Read the model definition and answer for the solid it produces. Units are mm, in the model's axes. Face numbers are marked on the shaded views. A direction names the side the tool comes from. Give positions to 0.01 mm unless a question says otherwise; leave off trailing zeros. Order: outer loops, then holes, each group sorted by start corner. A loop starts at its lowest first (then second) coordinate and runs counter-clockwise, first axis right, second up.
Autodesk Inventor part; units mm, degrees
ref_plane "Work Plane1" through (-2.5, 0, 0) normal (1, 0, 0) x (0, 1, 0)
ref_plane "XZ Plane" through (0, 0, 0) normal (0, 1, 0) x (-1, 0, 0)
ref_plane "XY Plane" through (0, 0, 0) normal (0, 0, 1) x (1, 0, 0)
sketch "Sketch1" plane through (0, 0, 0) normal (0, 0, 1) x (1, 0, 0)
  circle A0 centre (0, 0) radius 2
  circle A1 centre (0, 0) radius 6
  dimension "d0" = 4
  dimension "d1" = 12
extrude "Extrusion1" add sketch "Sketch1" along normal blind 5
ref_plane "Work Plane1" through (-2.5, 0, 0) normal (1, 0, 0) x (0, 1, 0)
sketch "Sketch5" plane through (-2.5, 0, 0) normal (1, 0, 0) x (0, 1, 0)
  line L0 (2.5, 0) -> (-2.5, 0)
  line L1 (-2.5, 0) -> (-2.5, 5)
  line L2 (-2.5, 5) -> (2.5, 5)
  line L3 (2.5, 5) -> (2.5, 0)
  point P0 (0, 0)
  point P1 (0, 0)
  dimension "d5" = 5
  dimension "d6" = 5
extrude "Extrusion2" add sketch "Sketch5" against normal blind 6
sketch "Sketch7" plane through (-8.5, 0, 0) normal (-1, 0, 0) x (0, 0, 1)
  line L0 (0, 2.5) -> (0, -2.5)
  line L1 (0, -2.5) -> (5, -2.5)
  line L2 (5, -2.5) -> (5, 2.5)
  line L3 (5, 2.5) -> (0, 2.5)
  point P0 (0, 0)
extrude "Extrusion3" add sketch "Sketch7" along normal blind 17
sketch "Sketch8" plane through (0, 0, 5) normal (0, 0, 1) x (1, 0, 0)
  line L0 (-25.5, 5) -> (-25.5, -5)
  line L1 (-25.5, -2.5) -> (-25.5, 2.5)
  line L2 (-6.5, 3.5) -> (-6.5, -3.5)
  arc A0 (-25.5, 5) -> (-6.5, 3.5) centre (7.5988, 303.1685) ccw
  arc A1 (-6.5, -3.5) -> (-25.5, -5) centre (7.5988, -303.1685) ccw
  point P0 (0, 0)
  point P1 (-25.5, 0)
  point P2 (-25.5, 0)
  point P3 (-6.5, 0)
  dimension "d11" = 10
  dimension "d12" = 7
  dimension "d13" = 6.5
  dimension "d14" = 300
  dimension "d15" = 300
extrude "Extrusion4" add sketch "Sketch8" against normal blind 6 and the other way blind 1
sketch "Sketch9" plane through (-5.4544, 2.5, 5) normal (0, 1, 0) x (1, 0, 0)
  line L0 (-20.0456, 7.5) -> (-20.0456, -2.5) construction
  line L1 (-20.0456, -1) -> (-20.0456, 6)
  line L2 (-1.0456, 6) -> (-1.0456, -1)
  arc A0 (-20.0456, 7.5) -> (-1.0456, 6) centre (13.0532, 305.6685) ccw
  arc A1 (-1.0456, -1) -> (-20.0456, -2.5) centre (13.0532, -300.6685) ccw
  line L3 (-1.0456, 6) -> (-1.0456, -1)
  line L4 (-20.0456, 6) -> (-1.0456, 6)
  line L5 (-20.0456, -1) -> (-1.0456, -1)
  line L6 (-20.0456, 6) -> (-20.0456, 7.5)
  line L7 (-20.0456, -2.5) -> (-20.0456, -1)
  point P0 (5.4544, 5)
  point P1 (-20.0456, 2.5)
  dimension "d20" = 10
  dimension "d21" = 300
  dimension "d22" = 300
extrude "Extrusion5" add sketch "Sketch9" along normal blind 2.5 and the other way blind 7.5 contours L5 A1 L7 | L6 A0 L4
sketch "Sketch10" plane through (-25.5, 5, -1) normal (0, 0, 1) x (1, 0, 0)
  arc A0 (0, 0) -> (19, -1.5) centre (33.0988, 298.1685) ccw
  line L0 (19, -1.5) -> (19, 0)
  line L1 (0, 0) -> (19, 0)
  arc A1 (19, -8.5) -> (0, -10) centre (33.0988, -308.1685) ccw
  line L2 (19, -10) -> (0, -10)
  line L3 (19, -10) -> (19, -8.5)
  point P0 (25.5, -5)
extrude "Extrusion6" cut sketch "Sketch10" along normal through all both and the other way through all
fillet "Fillet1" radius 2 4 edges at (-16.0467, 4.1018, 6.6018) (-16.0467, 4.1018, -1.6018) (-16.0467, -4.1018, 6.6018) (-16.0467, -4.1018, -1.6018)
sketch "Sketch11" plane through (-25.5, 0, 0) normal (-1, 0, 0) x (0, 0, 1)
  circle A0 centre (2.5, 0) radius 1.5
  line L0 (5.5122, 5) -> (-0.5122, 5)
  line L1 (7.5, 3.0122) -> (7.5, -3.0122)
  point P0 (0, 0)
  point P1 (7.5, 0)
  point P2 (2.5, 5)
  dimension "d30" = 3
extrude "Extrusion7" cut sketch "Sketch11" against normal blind 10
properties part number "Arm2" material "ABS Plastic"
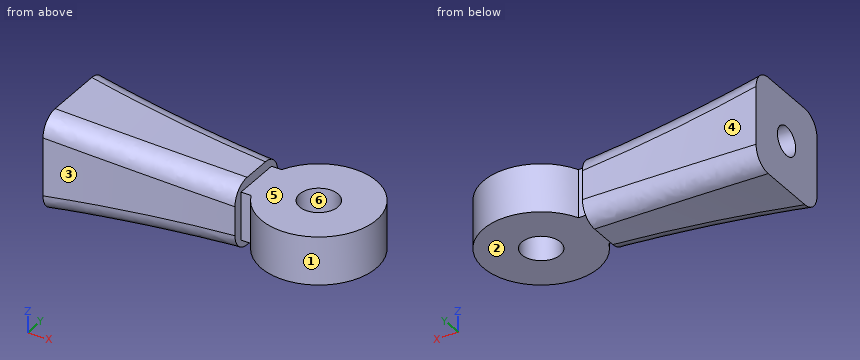
1) The part is cut by section B-B on y = 0. Determine the outline of the cut face in (x, z), and give its area (3 significant figures).
Final values:
outline: (-25.5, -2.5) arc R300 cw to (-6.5, -1) - (-6.5, 0) - (-2, 0) - (-2, 5) - (-6.5, 5) - (-6.5, 6) arc R300 cw to (-25.5, 7.5) - (-25.5, 4) - (-15.5, 4) - (-15.5, 1) - (-25.5, 1) - close; (2, 0) - (6, 0) - (6, 5) - (2, 5) - close
area: 170 mm2
2) The part is cut by section C-C on z = 2.5. Determine the outline of the cut face in (x, y), and give its area (3 significant figures).
Final values:
outline: (-25.5, -5) arc R300 cw to (-6.5, -3.5) - (-6.5, -2.5) - (-5.45, -2.5) arc R6 ccw (long way) to (-5.45, 2.5) - (-6.5, 2.5) - (-6.5, 3.5) arc R300 cw to (-25.5, 5) - (-25.5, 1.5) - (-15.5, 1.5) - (-15.5, -1.5) - (-25.5, -1.5) - close; hole circle Ø4 at (0, 0)
area: 232 mm2
3) The part is cut by section D-D on x = -6. Determine the outline of the cut face in (y, z).
Final values:
outline: (-2.5, 0) - (2.5, 0) - (2.5, 5) - (-2.5, 5) - close
4) For a pull along Y with two mould halves and no side action, classify the marked faces 4, 5 and 6 as released by +Y, released by -Y, zero draft, split by the parting line, or undercut.
Final values:
face 4: released by +Y
face 5: zero draft
face 6: undercut
5) A tool of negligible diameter and unlimited length cuts with its end or side. For the marked faces 1, 2 and 3, from which of +Z, -Z, +X, -X, +Y, -Y can it reach the whole face along a straight path? Write none if from no direction.
Final values:
face 1: +Z, -Z
face 2: -Z, +X, +Y, -Y
face 3: +Z, -Z, -Y
6) Consider L1, parallel to Y at x = 0, z = 2.25; L2, parallel to Y at x = -21.75, z = 2.5; L3, parallel to X at y = 1, z = 0.5. Determine where each line is inside the solid, lowest interval first.
Final values:
L1: y = -6 to -2, 2 to 6
L2: y = -4.61 to -1.5, 1.5 to 4.61
L3: x = -25.5 to -1.73, 1.73 to 5.92
7) The part is cut by section A-A on x = 0. Determine the outline of the cut face in (y, z), and give its area (3 significant figures).
Final values:
outline: (-6, 0) - (-2, 0) - (-2, 5) - (-6, 5) - close; (2, 0) - (6, 0) - (6, 5) - (2, 5) - close
area: 40.0 mm2
8) Given pin 1 (3.5 mm diameter, centred on y = 0, z = 2.5, fed in from -X); pin 2 (6 mm diameter, centred on x = 2, y = 3, fed in from +Z); pin 3 (3 mm diameter, centred on x = -22, z = 5.5, fed in from -Y); pin 4 (6 mm diameter, centred on x = -19, y = 2, fed in from +Z), each flat-ended and moving along its own axis, determine where each tip first touches the part or whether it passes through.
Final values:
pin 1: stops at x = -25.5
pin 2: stops at z = 5
pin 3: stops at y = -4.78
pin 4: stops at z = 7.13
